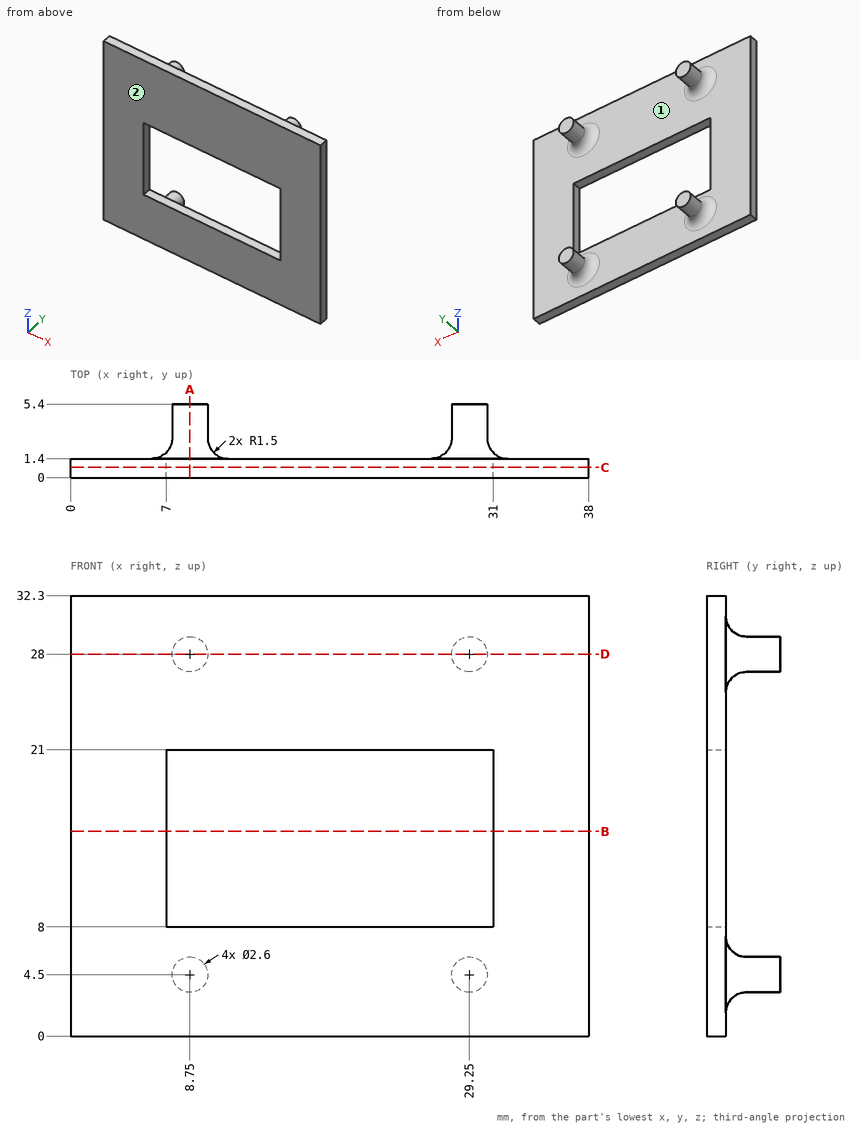
Job drawing, mm, ordinate dimensions from the low corner. One solid piece. Coordinates: 2 decimals unless noted, no trailing zeros. Order: outer loops, then holes, each group sorted by start corner. A loop starts at its lowest first (then second) coordinate and runs counter-clockwise, first axis right, second up. Notation, with made-up numbers: M 1,71 L 48,71 A23 ccw 48,107 Z; hole C -3,20.25 d6. An arc over 180 degrees is marked long. One line per question, with ' | ' between items.
Q1. Slice it at C-C (y = 0.75). Give the cut face in (x, z), and give its area (3 significant figures).
A:
outline: M 0,0 L 38,0 L 38,32.3 L 0,32.3 Z; hole M 7,8 L 31,8 L 31,21 L 7,21 Z | area: 915 mm^2
Q2. Pin check, flat tips, straight feed: P1, Ø2, axis at y = 3.5, z = 16.5, coming from the +X side; P2, Ø2, axis at x = 28.5, z = 21, coming from the +Y side. Stop position of each tip, or through.
A:
P1: passes through | P2: stops at y = 1.4
Q3. Two-plate mould, pull along X, no slides. Class the marked faces 1 and 2: +X half, -X half, draft (parallel to the pull), parting line (faces both ways), or undercut.
A:
face 1: undercut | face 2: draft
Q4. Slice it at A-A (x = 8.75). Give the cut face in (y, z).
A:
outline: M 0,0 L 1.4,0 L 1.4,1.7 A1.5 cw 2.9,3.2 L 5.4,3.2 L 5.4,5.8 L 2.9,5.8 A1.5 cw 1.4,7.3 L 1.4,8 L 0,8 Z; M 0,21 L 1.4,21 L 1.4,25.2 A1.5 cw 2.9,26.7 L 5.4,26.7 L 5.4,29.3 L 2.9,29.3 A1.5 cw 1.4,30.8 L 1.4,32.3 L 0,32.3 Z
Q5. Drill centre lines: line 1 (X direction, y = 0.9, z = 15.5); line 2 (Z direction, x = 15.5, y = 0.7); line 3 (Y direction, x = 26, z = 3.5). Where is each one in solid material? Low to high.
A:
line 1: x = 0 to 7, 31 to 38 | line 2: z = 0 to 8, 21 to 32.3 | line 3: y = 0 to 1.4
Q6. Slice it at D-D (z = 28). Give the cut face in (x, y), and give its area (3 significant figures).
A:
outline: M 0,0 L 38,0 L 38,1.4 L 32.05,1.4 A1.5 cw 30.55,2.9 L 30.55,5.4 L 27.95,5.4 L 27.95,2.9 A1.5 cw 26.45,1.4 L 11.55,1.4 A1.5 cw 10.05,2.9 L 10.05,5.4 L 7.45,5.4 L 7.45,2.9 A1.5 cw 5.95,1.4 L 0,1.4 Z | area: 75.9 mm^2
Q7. Slice it at B-B (z = 15). Give the cut face in (x, y).
A:
outline: M 0,0 L 7,0 L 7,1.4 L 0,1.4 Z; M 31,0 L 38,0 L 38,1.4 L 31,1.4 Z
